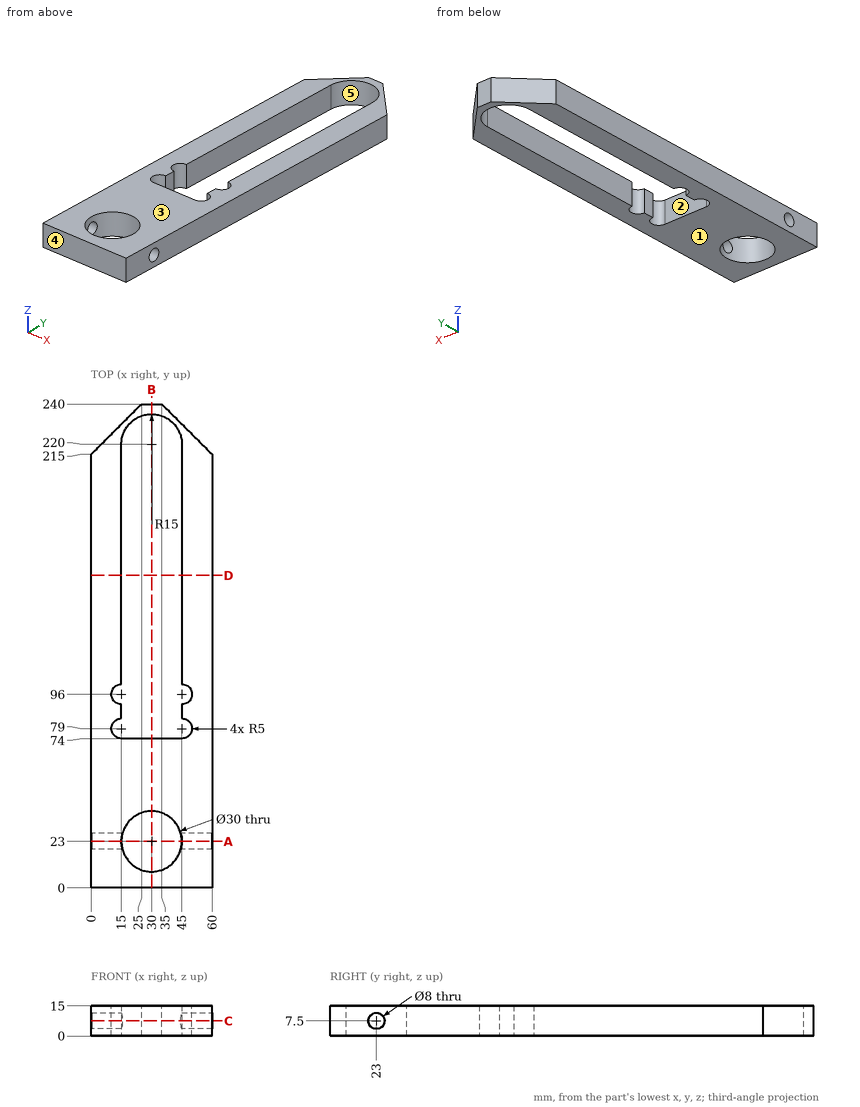
Check sheet for the drawn part. Datum: minimum x, y, z corner. Units: mm. A direction names the side the tool comes from. Give positions to 0.01 mm unless a question says otherwise; leave off trailing zeros. Order: outer loops, then holes, each group sorted by start corner. A loop starts at its lowest first (then second) coordinate and runs counter-clockwise, first axis right, second up. Notation, with made-up numbers: (79.5, 86.5) -> (126.5, 86.5) arc R25 cw to (126.5, 107.5) -> close; hole circle Ø9 at (-25.75, 11.5). An arc over 180 degrees is marked (long way). Use a Markdown table: item, result.
1) Depth check by flat-ended pin: pin 1 Ø5 at (x, z) = (13, 6.5) entering from +Y; pin 2 Ø6 at (x, z) = (8.5, 3) entering from -Y; pin 3 Ø8 at (x, z) = (20, 4.5) entering from +Y. Enter the tip coordinate at first touch or a pass-through.
Results:
| item | result |
|---|---|
| pin 1 | y = 230.5 |
| pin 2 | y = 0 |
| pin 3 | y = 239 |
2) Tool access check on the marked faces 1 and 2. Record the directions out of +Z, -Z, +X, -X, +Y, -Y that give a thin tool (end or side, any length) a straight path to the whole face; none if there is none.
Results:
| item | result |
|---|---|
| face 1 | -Z, +X, -X, +Y, -Y |
| face 2 | +Z, -Z |
3) Section check D-D, the plane y = 155. Record the boundary of the cut face in (x, z), then the cut area to 3 significant figures.
Results:
| item | result |
|---|---|
| outline | (0, 0) -> (15, 0) -> (15, 15) -> (0, 15) -> close; (45, 0) -> (60, 0) -> (60, 15) -> (45, 15) -> close |
| area | 450 mm² |
4) Mould release check, pull along Y, two halves, no side actions. Record for the marked faces 3, 4 and 5: pulls with the +Y half, pulls with the -Y half, needs draft (parallel to the pull), parting line crosses it, or undercut.
Results:
| item | result |
|---|---|
| face 3 | needs draft |
| face 4 | pulls with the -Y half |
| face 5 | undercut |
5) Material ranges on probe 1 along Y at (x, z) = (30, 7.75); probe 2 along Z at (x, y) = (52.5, 23); probe 3 along X at (y, z) = (179, 3.25), recorded low to high.
Results:
| item | result |
|---|---|
| probe 1 | 0 to 8, 38 to 74, 235 to 240 |
| probe 2 | 0 to 3.5, 11.5 to 15 |
| probe 3 | 0 to 15, 45 to 60 |
6) Section check B-B, the plane x = 30. Record the boundary of the cut face in (y, z).
Results:
| item | result |
|---|---|
| outline | (0, 0) -> (8, 0) -> (8, 15) -> (0, 15) -> close; (38, 0) -> (74, 0) -> (74, 15) -> (38, 15) -> close; (235, 0) -> (240, 0) -> (240, 15) -> (235, 15) -> close |
7) Section check C-C, the plane z = 7.5. Record the boundary of the cut face in (x, y), then the cut area to 3 significant figures.
Results:
| item | result |
|---|---|
| outline | (0, 0) -> (60, 0) -> (60, 19) -> (44.46, 19) arc R15 cw to (15.54, 19) -> (0, 19) -> close; (0, 27) -> (15.54, 27) arc R15 cw to (44.46, 27) -> (60, 27) -> (60, 215) -> (35, 240) -> (25, 240) -> (0, 215) -> close; hole (15, 74) -> (45, 74) arc R5 ccw to (45, 84) -> (45, 91) arc R5 ccw to (45, 101) -> (45, 220) arc R15 ccw to (15, 220) -> (15, 101) arc R5 ccw to (15, 91) -> (15, 84) arc R5 ccw to start |
| area | 7,930 mm² |
8) Section check A-A, the plane y = 23. Record the boundary of the cut face in (x, z), then the cut area to 3 significant figures.
Results:
| item | result |
|---|---|
| outline | (0, 0) -> (15, 0) -> (15, 3.5) -> (0, 3.5) -> close; (0, 11.5) -> (15, 11.5) -> (15, 15) -> (0, 15) -> close; (45, 0) -> (60, 0) -> (60, 3.5) -> (45, 3.5) -> close; (45, 11.5) -> (60, 11.5) -> (60, 15) -> (45, 15) -> close |
| area | 210 mm² |
